from build123d import *

# Parameters (mm, degrees)
F7_R      = 1.5
F10_DEPTH = 17.530616906
F8_R      = 1.5
F11_DEPTH = 17.530616906
F9_R      = 1.5
F12_DEPTH = 17.5306169047


with BuildPart() as f1:
    # F0 (on Right) → F1 (revolve)
    with BuildSketch(Plane.YZ):
        Polygon((-55.5, 0), (-45.5, 0), (-45.5, 2.1), (-38, 5), (-38, 12.7), (0, 12.7), (0, 20), (-55.5, 20), align=None)
    revolve(axis=Axis((0, 0, -2.8341766447), (0, 0, -1)))

    # F7 (on line) → F10 (cut, through all)
    with BuildSketch(Plane(origin=(48.06440991, 27.75, 0), x_dir=(-0.5, 0.8660254038, 0), z_dir=(0.8660254038, 0.5, 0))):
        with Locations((0, 8.85)):
            Circle(F7_R)
    extrude(amount=-F10_DEPTH, mode=Mode.SUBTRACT)

    # F8 (on line) → F11 (cut, through all)
    with BuildSketch(Plane(origin=(-48.06440991, 27.75, 0), x_dir=(-0.5, -0.8660254038, 0), z_dir=(-0.8660254038, 0.5, 0))):
        with Locations((0, 8.85)):
            Circle(F8_R)
    extrude(amount=-F11_DEPTH, mode=Mode.SUBTRACT)

    # F9 (on line) → F12 (cut, through all)
    with BuildSketch(Plane.XZ.offset(55.5)):
        with Locations((0, 8.85)):
            Circle(F9_R)
    extrude(amount=-F12_DEPTH, mode=Mode.SUBTRACT)


solid = f1.part
The model under review builds one solid part; all positions refer to its coordinate system, in mm. A direction names the side the tool comes from. Round coordinates to 2 decimals unless told otherwise and drop trailing zeros. Write each loop counter-clockwise with the first axis right and the second up, starting at its lowest first coordinate (ties: lowest second). Pieces come first, ordered by that corner, then holes. Notation, with made-up numbers: M 33.25,-31 L 81.25,-31 A15 cw 81.25,-11 Z; hole C -23.75,-8 d4. An arc over 180 degrees is marked long. Answer as CSV lines item,"result". Start each with the question number.
Q1. Wall thickness on line 1 along X through (y, z) = (0, 10); line 2 along Y through (x, z) = (0, 1.05): over which ranges is each line inside the solid? List them lowest first.
Q2. Clearance check with flat-ended pins moving along their axes: P1, Ø5, axis at x = -9, y = -41, coming from the -Z side; P2, Ø2, axis at x = -29, z = 6.5, coming from the -Y side; P3, Ø3, axis at x = -5.5, z = 7, coming from the -Y side. State where each tip first meets the part, or that it passes through.
Q3. Consider section C-C, the plane y = 0. Give the boundary of the cut face in (x, z), then the cut area to 3 significant figures.
Q4. Consider section B-B, the plane z = 8.85. Give the boundary of the cut face in (x, y).
Q5. The part is to be moulded in two halves that separate along Y. For faces 1 (the face through (-16.671, -52.937, 9.86)), 2 (the face through (-0.195, -46.858, 10.337)), 3 (the face through (-1.69, 38.33, 4.86)), 4 (the face through (-41.3, 22.19, 9.3)), say which applies: +Y half, -Y half, draft (parallel to the pull), parting line (faces both ways), or undercut.
Q6. Consider section A-A, the plane x = 0. Give the boundary of the cut face in (y, z), then the cut area to 3 significant figures.
Q7. Tool access review of faces 5 (the face through (27.686, 36.107, 1.065)), 6 (the face through (40.177, 24.127, 10.115)): name each direction out of +Z, -Z, +X, -X, +Y, -Y from which nothing blocks a thin tool from reaching the whole face with its end or side.
Result set:
1,line 1,"x = -55.5 to -38, 38 to 55.5"
1,line 2,"y = -55.5 to -45.5, 45.5 to 55.5"
2,P1,"stops at z = 2.5"
2,P2,"stops at y = -47.92"
2,P3,"stops at y = -55.36"
3,outline,"M -55.5,0 L -45.5,0 L -45.5,2.1 L -38,5 L -38,12.7 L 38,12.7 L 38,5 L 45.5,2.1 L 45.5,0 L 55.5,0 L 55.5,20 L -55.5,20 Z"
3,area,"1,200 mm²"
4,outline,"M -48.8,26.44 A55.5 ccw -1.5,-55.48 L -1.5,-37.97 A38 cw -33.63,17.69 Z; M -47.3,29.04 L -32.13,20.28 A38 cw 32.13,20.28 L 47.3,29.04 A55.5 ccw Z; M 1.5,-55.48 A55.5 ccw 48.8,26.44 L 33.63,17.69 A38 cw 1.5,-37.97 Z"
5,face 1,"parting line"
5,face 2,"draft"
5,face 3,"undercut"
5,face 4,"undercut"
6,outline,"M -55.5,0 L -45.5,0 L -45.5,2.1 L -38,5 L -38,7.35 L -55.5,7.35 Z; M -55.5,10.35 L -38,10.35 L -38,12.7 L 38,12.7 L 38,5 L 45.5,2.1 L 45.5,0 L 55.5,0 L 55.5,20 L -55.5,20 Z"
6,area,"1,150 mm²"
7,face 5,"-Z"
7,face 6,"none"
